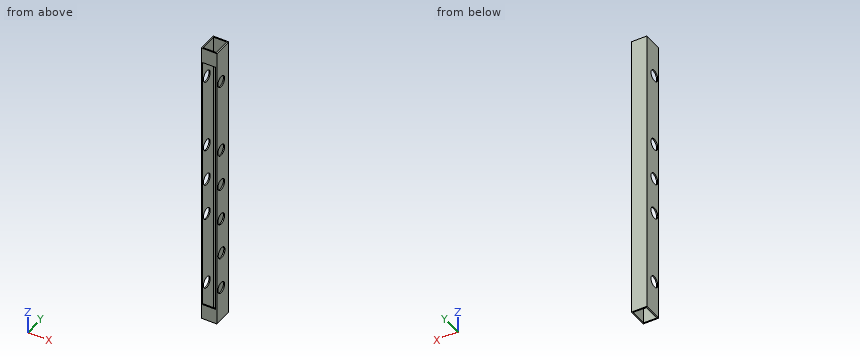
Autodesk Inventor part; units mm, degrees
ref_plane "Start Plane" through (0, 0, 25) normal (0, 0, 1) x (1, 0, 0)
ref_plane "End Plane" through (0, 0, 775) normal (0, 0, 1) x (1, 0, 0)
ref_plane "Work Plane5" through (628, -25, 25) normal (0, 0, -1) x (-1, 0, 0)
ref_plane "Start Plane" through (0, 0, 25) normal (0, 0, 1) x (1, 0, 0)
ref_plane "End Plane" through (0, 0, 775) normal (0, 0, 1) x (1, 0, 0)
sketch "Sketch" plane through (0, 0, 0) normal (0, 0, 1) x (1, 0, 0)
  line L0 (-20, -25) -> (20, -25)
  line L1 (20, -25) -> (20, 25)
  line L2 (20, 25) -> (-20, 25)
  line L3 (-20, 25) -> (-20, -25)
  line L4 (-20, -25) -> (20, 25) construction
  line L5 (20, -25) -> (-20, 25) construction
  line L6 (-17, 22) -> (17, 22)
  line L7 (17, 22) -> (17, -22)
  line L8 (17, -22) -> (-17, -22)
  line L9 (-17, -22) -> (-17, 22)
  point P0 (0, 0)
  dimension "Width" = 40
  dimension "Height" = 50
  dimension "Thickness" = 3
extrude "Body" add sketch "Sketch" along normal up to surface (750 mm away) from surface at 25
sketch "Sketch2" plane through (0, 0, 0) normal (0, 0, 1) x (1, 0, 0)
  line L0 (0, 0) -> (10, 0)
ref_plane "Work Plane3" through (0, 0, 0) normal (0, -1, 0) x (1, 0, 0)
sketch "Sketch3" plane through (0, 0, 0) normal (0, -1, 0) x (1, 0, 0)
  line L0 (-28, 25) -> (28, 25)
  line L1 (-28, 775) -> (28, 775)
  dimension "d10" = 750
ref_plane "Work Plane5" through (628, -25, 25) normal (0, 0, -1) x (-1, 0, 0)
split "Split2" plane through (628, -25, 25) removes the side toward (0, 0, -1)
ref_plane "Work Plane6" through (-72, -25, 775) normal (0, 0, 1) x (1, 0, 0)
split "Split3" plane through (-72, -25, 775) removes the side toward (0, 0, 1)
sketch "Sketch4" plane through (-20, -25, 775) normal (-1, 0, 0) x (0, 0, 1)
  line L0 (-750, 50) -> (0, 50)
  line L1 (-750, 0) -> (0, 0)
  line L2 (-660.75, 18.2875) -> (-89.25, 18.2875)
  line L3 (-750, 3) -> (-750, 47) construction
  line L4 (-750, 25) -> (0, 25) construction
  line L5 (0, 3) -> (0, 47) construction
  line L6 (-750, 0) -> (-750, 50)
  line L7 (0, 0) -> (0, 50)
  point P0 (-775, 25)
  point P1 (-375, 18.2875)
  point P2 (-375, 0)
  dimension "d11" = 571.5
  dimension "d44" = 18.2875
hole "Hole1" at (-20, -6.7125, 114.25) direction (1, 0, 0) diameter 28.575 end through all
pattern_linear "Rectangular Pattern1" count 3 spacing 285.75 along (0, 0, 1) of "Hole1"
sketch "Sketch5" plane through (-20, -25, 775) normal (-1, 0, 0) x (0, 0, 1)
  line L0 (0, 0) -> (0, 50)
  line L1 (-750, 50) -> (0, 50)
  line L2 (-750, 0) -> (-750, 50)
  line L3 (-750, 0) -> (0, 0)
  line L4 (-775, 25) -> (25, 25)
  point P0 (-375, 17)
  point P1 (-375, 19.9091)
  point P2 (-375, 25)
  point P3 (-375, 25)
  dimension "d35" = 8
hole "Hole2" [suppressed]
sketch "Sketch7" plane through (-20, -25, 775) normal (-1, 0, 0) x (0, 0, 1)
  line L0 (-666.5, 21) -> (-83.5, 21) construction
  line L1 (-766.8103, 25) -> (25, 25) construction
  point P0 (-375, 21)
  point P1 (-375, 25)
  dimension "d36" = 583
  dimension "d40" = 4
pattern_linear "Rectangular Pattern2" count 4 spacing 190.5 along (0, 0, 1) of "Hole1"
sketch "Sketch9" plane through (20, -25, 775) normal (1, 0, 0) x (0, 0, -1)
  line L0 (0, 50) -> (750, 50)
  line L1 (750, 0) -> (750, 50)
  line L2 (0, 50) -> (750, 50)
  line L3 (0, 0) -> (0, 50)
  line L4 (0, 0) -> (750, 0)
  circle A0 centre (660.8, 18.2875) radius 12.7
  circle A1 centre (279.75, 18.2875) radius 14.2875
  circle A2 centre (470.25, 18.2875) radius 14.2875
  circle A3 centre (660.75, 18.2875) radius 14.2875
  circle A4 centre (375, 18.2875) radius 14.2875
  circle A5 centre (89.25, 18.2875) radius 14.2875
  point P0 (775, 25)
  point P1 (565.5644, 19.942)
  dimension "d57" = 95.25
  dimension "d58" = 30.058
hole "Hole4" at (20, -5.058, 209.4356) direction (-1, 0, 0) diameter 28.575 depth 10
sketch "Sketch12" plane through (17, -25, 775) normal (-1, 0, 0) x (0, 0, 1)
  point P0 (-775, 25)
sketch "Sketch13" plane through (-20, -25, 775) normal (0, -1, 0) x (1, 0, 0)
  line L0 (0, -750) -> (0, 0)
  line L1 (3, -750) -> (3, 0)
  line L2 (37, -750) -> (37, 0)
  line L3 (-55, -750) -> (645, -750)
  line L4 (-55, 0) -> (645, 0)
  line L5 (37, -750) -> (37, 0)
  line L6 (3, -710.75) -> (37, -710.75)
  line L7 (37, -710.75) -> (37, -39.25)
  line L8 (37, -39.25) -> (3, -39.25)
  line L9 (3, -39.25) -> (3, -710.75)
  point P0 (20, -775)
  point P1 (37, -375)
  point P2 (37, -375)
  point P3 (37, -39.25)
  point P4 (3, -39.25)
  point P5 (37, -710.75)
  dimension "d73" = 671.5
extrude "Extrusion4" cut sketch "Sketch13" against normal blind 10 contours L1 L8 L2 L6
sketch "Sketch14" plane through (20, -25, 775) normal (1, 0, 0) x (0, 0, -1)
  circle A0 centre (375, 18.2875) radius 14.2875
  point P0 (775, 25)
equation "\"d22\" = Wheel_Seperation"
equation "\"d36\" = 3 * Wheel_Seperation2"
equation "\"d40\" = Wheel_HeightOffset2"
equation "\"d43\" = Wheel_MaxSeperation2"
equation "\"G_OFFSET_START\" = -25"
equation "\"G_OFFSET_END\" = -25"
equation "\"d5\" = -G_OFFSET_START"
equation "\"d6\" = Length + G_OFFSET_END"
equation "\"G_L\" = 750"
equation "\"Chassi_CentreDrop\" = 4"
equation "\"WheelBay_Depth\" = 55"
equation "\"Wheel_Diametre\" = 152.4"
equation "\"Wheel_Seperation\" = 285.75"
equation "\"Wheel_HeightOffset\" = 4"
equation "\"Wheel_Clearance\" = 13.05"
equation "\"Chassi_GroundClearance\" = 10.116"
equation "\"Wheel_CentreDrop\" = 4"
equation "\"Wheel_Seperation2\" = 194.33333"
equation "\"Wheel_Diametre2\" = 101.6"
equation "\"Wheel_HeightOffset2\" = 4"
equation "\"Wheel_Clearance2\" = 32.7"
equation "\"Chain_Pitch\" = 9.525"
equation "\"Wheel_MaxSeperation\" = 285.75"
equation "\"Wheel_CCSpan\" = 571.5"
equation "\"Wheel_CCSpan2\" = 471.5"
equation "\"Wheel_MaxSeperation2\" = 190.5"
equation "\"MotorholeCC\" = 95.25"
equation "\"MotorholeHorizontal\" = 95.01318"
equation "\"OutputshaftTopOffset\" = 30.058"
equation "\"Heightfromcenter\" = 6.7125"
equation "\"Chassi_SideRivetSpacing\" = 37.5"
equation "\"Sprocket_Thickness\" = 10.668"
equation "\"BumperMountingBarOffset\" = 177.8"
properties part number "50x40x3" material "Aluminum 6061"
Design review of the part built by this model. Coordinates are the model's own, in mm. Round coordinates to 2 decimals unless told otherwise and drop trailing zeros. Write each loop counter-clockwise with the first axis right and the second up, starting at its lowest first coordinate (ties: lowest second). Pieces come first, ordered by that corner, then holes. Notation, with made-up numbers: M 16,-27.5 L 36,-27.5 A31 ccw 36,0.5 Z; hole C -19.5,23 d4. An arc over 180 degrees is marked long. One line per item, written item: value. Start each with the question number.
1. Take a section at B-B on z = 685.75. State the section outline as (x, y) points (3 decimals).
2. To check wall thickness, follow probe 1 along X at (y, z) = (-17, 86.5); probe 2 along Y at (x, z) = (18, 114); probe 3 along Z at (x, y) = (-17.5, -2). State the ranges of each line that lie inside material, in increasing order. Write a range as from..to.
3. Clearance check with flat-ended pins moving along their axes: P1, Ø3, axis at x = 11, z = 429, coming from the -Y side; P2, Ø14, axis at y = 5.5, z = 305.5, coming from the +X side. State where each tip first meets the part, or that it passes through.
4. Take a section at C-C on z = 304. State the section outline as (x, y) points, then the cut area to 3 significant figures.
5. Take a section at A-A on x = 8. State the section outline as (y, z) points.
Computed:
1. outline: M -20,-25 L -17,-25 L -17,-21 L -20,-21 Z; M -20,7.575 L -17,7.575 L -17,22 L 17,22 L 17,7.575 L 20,7.575 L 20,25 L -20,25 Z; M 17,-25 L 20,-25 L 20,-21 L 17,-21 Z
2. probe 1: x = -20..-17, 17..20
2. probe 2: y = -25..-21, 7.57..25
2. probe 3: z = 25..100.76, 127.74..291.26, 318.24..386.51, 413.49..481.76, 508.74..672.26, 699.24..775
3. P1: stops at y = 22
3. P2: stops at x = 20
4. outline: M -20,-25 L -17,-25 L -17,-20.98 L -20,-20.98 Z; M -20,7.56 L -17,7.56 L -17,22 L 17,22 L 17,7.56 L 20,7.56 L 20,25 L -20,25 Z; M 17,-25 L 20,-25 L 20,-20.98 L 17,-20.98 Z
4. area: 231 mm²
5. outline: M -25,25 L -22,25 L -22,64.25 L -25,64.25 Z; M -25,735.75 L -22,735.75 L -22,775 L -25,775 Z; M 22,25 L 25,25 L 25,775 L 22,775 Z
